Build history of the part. All positions in model axes, mm. A direction names the side the tool comes from. Round coordinates to 2 decimals unless told otherwise and drop trailing zeros. Order: outer loops, then holes, each group sorted by start corner. A loop starts at its lowest first (then second) coordinate and runs counter-clockwise, first axis right, second up. Notation, with made-up numbers: M 66,-35 L 98,-35 A26 cw 98,-9 Z; hole C 1,-0.5 d9. An arc over 180 degrees is marked long. One line per item, written item: value. Start each with the question number.
Item 1: Tool access for faces 1 (the flat face through (0, 13, -692)), 2 (the flat face through (14, 3.175, -692)): list every direction of +Z, -Z, +X, -X, +Y, -Y with a clear straight run to the whole face (end or side of a thin tool).
Item 2: Band-saw the part on A-A, the plane z = -87.5. Write the cut outline in (x, y) (3 decimals).
Item 3: Probe L1, parallel to X at y = 1.85, z = -838.2; L2, parallel to X at y = 20.5, z = -262 (3 decimals). List the from-to ranges inside material, lowest first.
Item 4: Pin check, flat tips, straight feed: pin 1 (10 mm diameter, centred on x = 6.5, y = 20, fed in from +Z); pin 2 (5.5 mm diameter, centred on x = 12.7, z = -701.675, fed in from +Y) (3 decimals); pin 3 (3 mm diameter, centred on x = 12.7, z = -155.575, fed in from +Y); pin 4 (11 mm diameter, centred on y = 15, z = -784.5, fed in from +X) (3 decimals). Stop position of each tip, or through.
```python
from build123d import *

# Parameters (mm, degrees)
EXTRUDE1_DEPTH     = 1403.35
SKETCH2_R          = 2.4257
CUT_EXTRUDE2_DEPTH = 1404.809653229
LPATTERN1_COUNT    = 11
LPATTERN1_PITCH    = 136.525
FILLET1_R          = 12.7


with BuildPart() as part:
    # Sketch1 → Extrude1 (new body)
    with BuildSketch(Plane.XY):
        Polygon((0, 0), (25.4, 0), (25.4, 3.175), (3.175, 3.175), (3.175, 25.4), (0, 25.4), align=None)
    extrude(amount=-EXTRUDE1_DEPTH)

    # Sketch2 → Cut-Extrude2 (cut, through all)
    with BuildSketch(Plane(origin=(0, 0, 0), x_dir=(1, 0, 0), z_dir=(0, 1, 0))):
        with Locations(Location((12.7, 19.05, 0), (0, 0, 180))):
            Circle(SKETCH2_R)
    cut_extrude2 = extrude(amount=CUT_EXTRUDE2_DEPTH, mode=Mode.SUBTRACT)

    # LPattern1: Cut-Extrude2 ×11
    with Locations(*[(0, 0, -i * LPATTERN1_PITCH) for i in range(1, LPATTERN1_COUNT)]):
        add(cut_extrude2, mode=Mode.SUBTRACT)

    # Fillet1
    fillet1_edges = [part.edges().sort_by_distance(p)[0] for p in [
        (1.5875, 25.4, -1403.35),
        (1.5875, 25.4, 0),
    ]]
    fillet(fillet1_edges, radius=FILLET1_R)


solid = part.part
```
Output:
1. face 1: +Z, -Z, -X, +Y, -Y
1. face 2: +Z, -Z, +X, +Y
2. outline: M 0,0 L 25.4,0 L 25.4,3.175 L 3.175,3.175 L 3.175,25.4 L 0,25.4 Z
3. L1: x = 0 to 10.27, 15.13 to 25.4
3. L2: x = 0 to 3.175
4. pin 1: stops at z = -0.51
4. pin 2: stops at y = 3.175
4. pin 3: passes through
4. pin 4: stops at x = 3.175
